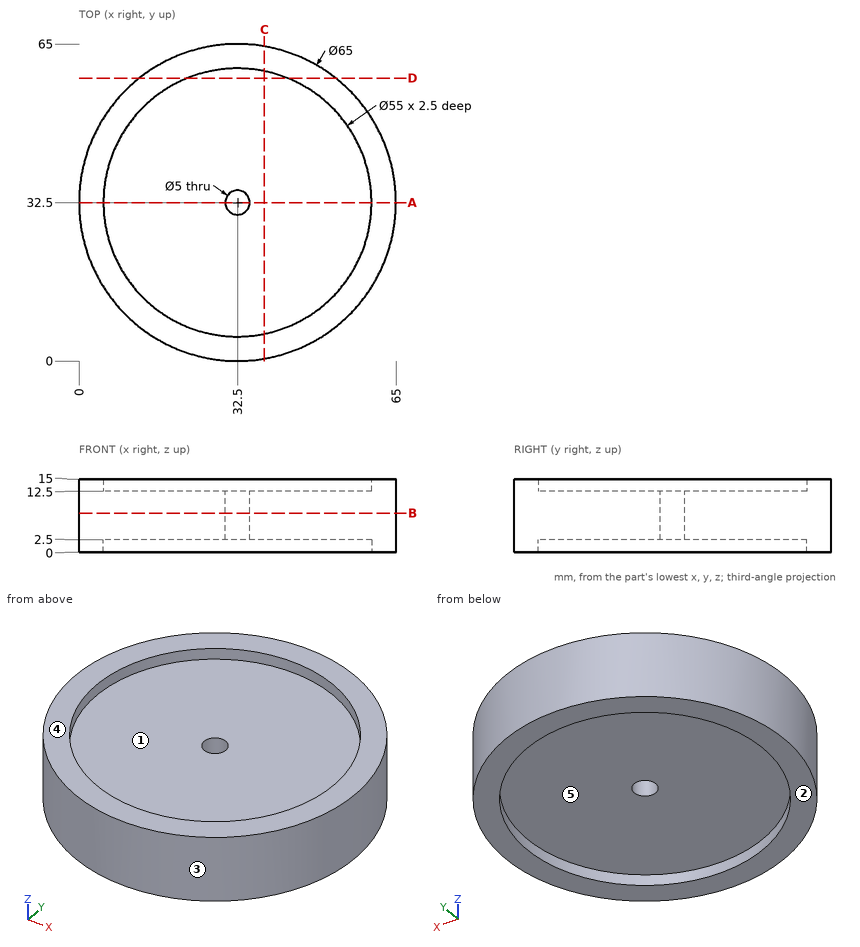
Print and shaded views of the part. All mm, measured from the part's lowest x, y and z. A direction names the side the tool comes from. Coordinates: 2 decimals unless noted, no trailing zeros. Order: outer loops, then holes, each group sorted by start corner. A loop starts at its lowest first (then second) coordinate and runs counter-clockwise, first axis right, second up. Notation, with made-up numbers: (-34.75, 84.25) -> (-20.75, 84.25) arc R24 ccw to (-20.75, 102.25) -> close; hole circle Ø6 at (83, 81). An arc over 180 degrees is marked (long way). Answer as a JSON object with one key per item and string values. Group by question number.
1) Flat gauge pins, fed straight in: pin 1 (4.5 mm diameter, centred on x = 32.5, y = 32.5, fed in from +Z); pin 2 (1 mm diameter, centred on y = 39.5, z = 2.5, fed in from +X); pin 3 (6 mm diameter, centred on x = 38.5, y = 50.5, fed in from +Z); pin 4 (2 mm diameter, centred on x = 36.5, y = 50.5, fed in from -Z). Where does each tip first touch, or does it go through?
2) Cut at A-A, the plane y = 32.5. Write the cut outline in (x, z), then the cut area to 3 significant figures.
3) Cut at C-C, the plane x = 38. Write the cut outline in (y, z).
4) Which spindle directions (+Z, -Z, +X, -X, +Y, -Y) get a long thin tool onto all of the face, cutting with end or side? Do the marked faces 1 and 2. Say none if no direction does.
5) Cut at D-D, the plane y = 58. Write the cut outline in (x, z).
6) Pull direction X, two halves, no side cores. Call the marked faces 3, 4 and 5: +X half, -X half, draft (parallel to the pull), parting line (faces both ways), or undercut.
7) Cut at B-B, the plane z = 8. Write the cut outline in (x, y), then the cut area to 3 significant figures.
8) Drill centre lines: L1, parallel to Y at x = 32.5, z = 1.85; L2, parallel to Y at x = 32.5, z = 7.5; L3, parallel to Z at x = 12, y = 21. Where is each one in solid material? Low to high.
Check values:
{
 "1": {"pin 1": "passes through", "pin 2": "stops at x = 64.34", "pin 3": "stops at z = 12.5", "pin 4": "stops at z = 2.5"},
 "2": {"outline": "(0, 0) -> (5, 0) -> (5, 2.5) -> (30, 2.5) -> (30, 12.5) -> (5, 12.5) -> (5, 15) -> (0, 15) -> close; (35, 2.5) -> (60, 2.5) -> (60, 0) -> (65, 0) -> (65, 15) -> (60, 15) -> (60, 12.5) -> (35, 12.5) -> close", "area": "650 mm²"},
 "3": {"outline": "(0.47, 0) -> (5.56, 0) -> (5.56, 2.5) -> (59.44, 2.5) -> (59.44, 0) -> (64.53, 0) -> (64.53, 15) -> (59.44, 15) -> (59.44, 12.5) -> (5.56, 12.5) -> (5.56, 15) -> (0.47, 15) -> close"},
 "4": {"face 1": "+Z", "face 2": "-Z, +X, -X, +Y, -Y"},
 "5": {"outline": "(12.35, 0) -> (22.2, 0) -> (22.2, 2.5) -> (42.8, 2.5) -> (42.8, 0) -> (52.65, 0) -> (52.65, 15) -> (42.8, 15) -> (42.8, 12.5) -> (22.2, 12.5) -> (22.2, 15) -> (12.35, 15) -> close"},
 "6": {"face 3": "parting line", "face 4": "draft", "face 5": "undercut"},
 "7": {"outline": "circle Ø65 at (32.5, 32.5); hole circle Ø5 at (32.5, 32.5)", "area": "3,300 mm²"},
 "8": {"L1": "y = 0 to 5, 60 to 65", "L2": "y = 0 to 30, 35 to 65", "L3": "z = 2.5 to 12.5"}
}
